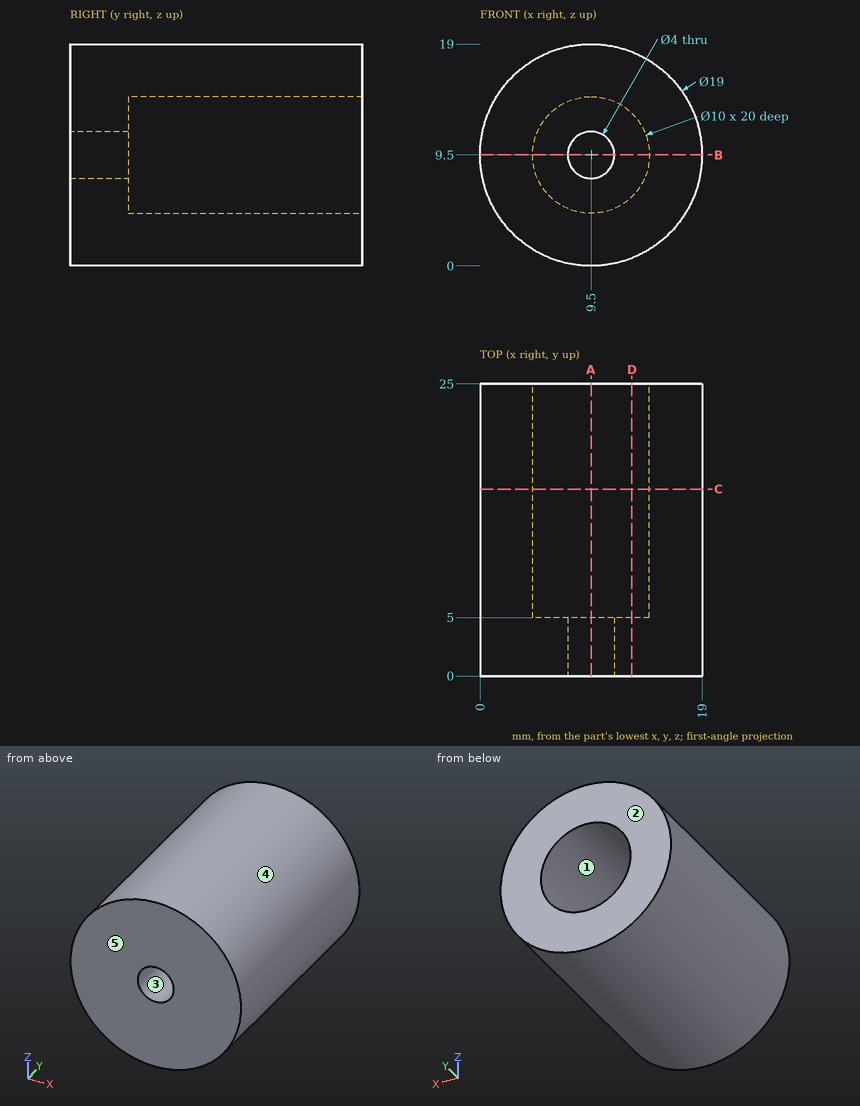
Verification items for this drawing (mm, ordinates from the low corner). A direction names the side the tool comes from. Coordinates: 2 decimals unless noted, no trailing zeros. Order: outer loops, then holes, each group sorted by start corner. A loop starts at its lowest first (then second) coordinate and runs counter-clockwise, first axis right, second up. Notation, with made-up numbers: (4.25, -30.5) - (22.25, -30.5) arc R24 ccw to (22.25, 7.5) - close; hole circle Ø10 at (83, 72.5). An arc over 180 degrees is marked (long way). Answer in a Markdown table with one row per item. Add a question column.
1. Section check C-C (y = 16). Enter the section's corners in (x, z).
2. Section check D-D (x = 13). Enter the section's corners in (y, z), plus the area to 3 significant figures.
3. Material ranges on L1, parallel to X at y = 18.5, z = 9.5; L2, parallel to X at y = 2.4, z = 9.5; L3, parallel to Y at x = 8.75, z = 5.5, recorded low to high. Write a range as [from, to].
4. Access from +Z, -Z, +X, -X, +Y, -Y to the whole of each face (thin tool, end or side, straight path). Record for the marked faces 1 and 2.
5. Gauge pin test, flat ends, axial feed: pin 1 Ø3 at (y, z) = (14, 4.5) entering from +X; pin 2 Ø8 at (x, z) = (7.5, 7.5) entering from +Y; pin 3 Ø1 at (x, y) = (11.5, 4) entering from +Z; pin 4 Ø8 at (y, z) = (10, 14) entering from -X. Record the tip position at first contact, or that the pin passes through.
6. Section check B-B (z = 9.5). Enter the section's corners in (x, y).
7. Section check A-A (x = 9.5). Enter the section's corners in (y, z), plus the area to 3 significant figures.
8. Draft check along X on the marked faces 3, 4 and 5. Enter one of: +X half, -X half, draft (parallel to the pull), parting line (faces both ways), or undercut.
Data:
| question | item | result |
|---|---|---|
| 1 | outline | circle Ø19 at (9.5, 9.5); hole circle Ø10 at (9.5, 9.5) |
| 2 | outline | (0, 0.67) - (25, 0.67) - (25, 5.93) - (5, 5.93) - (5, 13.07) - (25, 13.07) - (25, 18.33) - (0, 18.33) - close |
| 2 | area | 299 mm² |
| 3 | L1 | x = [0, 4.5], [14.5, 19] |
| 3 | L2 | x = [0, 7.5], [11.5, 19] |
| 3 | L3 | y = [0, 5] |
| 4 | face 1 | +Y |
| 4 | face 2 | +Z, -Z, +X, -X, +Y |
| 5 | pin 1 | stops at x = 18.33 |
| 5 | pin 2 | stops at y = 25 |
| 5 | pin 3 | stops at z = 18.88 |
| 5 | pin 4 | stops at x = 0.01 |
| 6 | outline | (0, 0) - (7.5, 0) - (7.5, 5) - (4.5, 5) - (4.5, 25) - (0, 25) - close; (11.5, 0) - (19, 0) - (19, 25) - (14.5, 25) - (14.5, 5) - (11.5, 5) - close |
| 7 | outline | (0, 0) - (25, 0) - (25, 4.5) - (5, 4.5) - (5, 7.5) - (0, 7.5) - close; (0, 11.5) - (5, 11.5) - (5, 14.5) - (25, 14.5) - (25, 19) - (0, 19) - close |
| 7 | area | 255 mm² |
| 8 | face 3 | undercut |
| 8 | face 4 | parting line |
| 8 | face 5 | draft |
